```python
from build123d import *

# Parameters (mm, degrees)
SKETCH1_R           = 609.6
SKETCH1_R_2         = 508
BOSS_EXTRUDE1_DEPTH = 12.7
SKETCH2_R           = 11
CUT_EXTRUDE1_DEPTH  = 12.7


with BuildPart() as part:
    # Sketch1 → Boss-Extrude1 (new body)
    with BuildSketch(Plane.XY):
        Circle(SKETCH1_R)
        Circle(SKETCH1_R_2, mode=Mode.SUBTRACT)
    extrude(amount=BOSS_EXTRUDE1_DEPTH)

    # Sketch2 → Cut-Extrude1 (cut)
    with BuildSketch(Plane.XY):
        with Locations((0, 215.685000111)):
            Circle(SKETCH2_R)
        with Locations((0, 558.8)):
            Circle(SKETCH2_R)
        with Locations((279.4, 483.934995635)):
            Circle(SKETCH2_R)
        with Locations((483.934995635, 279.4)):
            Circle(SKETCH2_R)
        with Locations((558.8, 0)):
            Circle(SKETCH2_R)
        with Locations((483.934995635, -279.4)):
            Circle(SKETCH2_R)
        with Locations((279.4, -483.934995635)):
            Circle(SKETCH2_R)
        with Locations((0, -558.8)):
            Circle(SKETCH2_R)
        with Locations((-279.4, -483.934995635)):
            Circle(SKETCH2_R)
        with Locations((-483.934995635, -279.4)):
            Circle(SKETCH2_R)
        with Locations((-558.8, 0)):
            Circle(SKETCH2_R)
        with Locations((-483.934995635, 279.4)):
            Circle(SKETCH2_R)
        with Locations((-279.4, 483.934995635)):
            Circle(SKETCH2_R)
    extrude(amount=CUT_EXTRUDE1_DEPTH, mode=Mode.SUBTRACT)


solid = part.part
```
The listing builds one solid part. Answer for the finished solid, in the listing's coordinates (mm). Round coordinates to 2 decimals unless told otherwise and drop trailing zeros. Loops run counter-clockwise (first coordinate to the right, second up) from the corner with the lowest first, then second, coordinate; pieces in that order, holes last. Notation, with made-up numbers: (70.5, 8.25) - (85.5, 8.25) arc R28 ccw to (85.5, 39.25) - close; hole circle Ø4 at (52, 52). An arc over 180 degrees is marked (long way). Use one line per item in the form item = value. Start each with the question number.
1. Given pin 1 Ø1.5 at (y, z) = (233, 11) entering from +X; pin 2 Ø4 at (y, z) = (-398.5, 8) entering from +X; pin 3 Ø4 at (y, z) = (-118, 7.5) entering from -X, each flat-ended and moving along its own axis, determine where each tip first touches the part or whether it passes through.
2. Consider line 1 (Y direction, x = 279.4, z = 5) (3 decimals); line 2 (Y direction, x = 278.5, z = 10.75); line 3 (X direction, y = -48, z = 3.5). Determine where each line is inside the solid, lowest interval first. Write a range as [from, to].
3. The part is cut by section C-C on z = 7.75. Give the number of separate pieces and of enclosed holes in the cut face, then the cut area to 3 significant figures.
4. For a pull along Y with two mould halves and no side action, classify faces 1 (the face through (-229, 454, 0)), 2 (the face through (-110.12, -495.92, 6.26)), 3 (the face through (-483.76, -370.93, 6.26)) as pulls with the +Y half, pulls with the -Y half, needs draft (parallel to the pull), parting line crosses it, or undercut.
5. The part is cut by section B-B on x = -210. Determine the outline of the cut face in (y, z).
6. The part is cut by section A-A on y = 433. Determine the outline of the cut face in (x, z), then the cut area to 3 significant figures.
Geometry check:
q1.pin_1 = 563.62
q1.pin_2 = 463.03
q1.pin_3 = -598.46
q2.line_1 = [-541.801, -494.935], [-472.935, -424.264], [424.264, 472.935], [494.935, 541.801]
q2.line_2 = [-542.26, -494.9], [-472.97, -424.85], [424.85, 472.97], [494.9, 542.26]
q2.line_3 = [-607.71, -505.73], [505.73, 607.71]
q3.separate_pieces = 1
q3.enclosed_holes = 13
q3.area = 352,000 mm^2
q4.face_1 = needs draft
q4.face_2 = undercut
q4.face_3 = parting line crosses it
q5.outline = (-572.29, 0) - (-462.56, 0) - (-462.56, 12.7) - (-572.29, 12.7) - close; (462.56, 0) - (572.29, 0) - (572.29, 12.7) - (462.56, 12.7) - close
q6.outline = (-429.1, 0) - (-265.66, 0) - (-265.66, 12.7) - (-429.1, 12.7) - close; (265.66, 0) - (429.1, 0) - (429.1, 12.7) - (265.66, 12.7) - close
q6.area = 4,150 mm^2
